Check sheet for the modelled part. Datum: model origin and axes. Units: mm. Give positions to 0.01 mm unless a question says otherwise; leave off trailing zeros. Write each loop counter-clockwise with the first axis right and the second up, starting at its lowest first coordinate (ties: lowest second). Pieces come first, ordered by that corner, then holes.
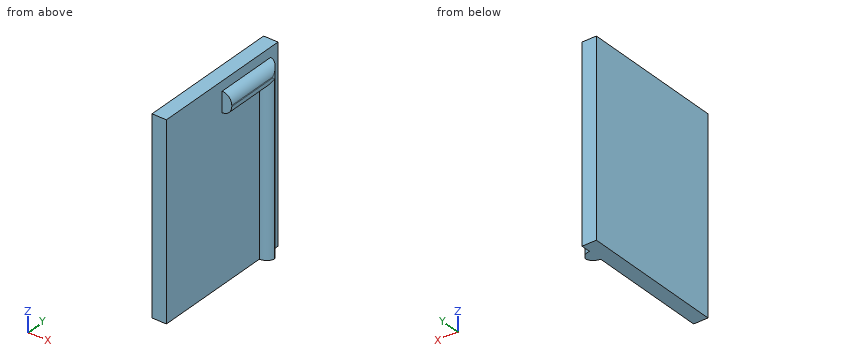
from build123d import *

# Parameters (mm, degrees)
SKETCH1_W           = 40
SKETCH1_H           = 30
BOSS_EXTRUDE1_DEPTH = 3
BOSS_EXTRUDE2_DEPTH = 2
FILLET1_R           = 2


with BuildPart() as part:
    # Sketch1 → Boss-Extrude1 (new body)
    with BuildSketch(Plane(origin=(0, 0, 0), x_dir=(0, 0, -1), z_dir=(1, 0, 0))):
        Rectangle(SKETCH1_W, SKETCH1_H)
    extrude(amount=BOSS_EXTRUDE1_DEPTH)

    # Sketch2 → Boss-Extrude2 (add)
    with BuildSketch(Plane(origin=(3, 0, 0), x_dir=(0, 0, -1), z_dir=(1, 0, 0))):
        Polygon((20, 10), (20, 13), (-13.768503326, 13), (-18, 13), (-18, 10), (-18, 0), (-13.768503326, 0), (-13.768503326, 10), align=None)
    extrude(amount=BOSS_EXTRUDE2_DEPTH)

    # Fillet1
    # the kernel refuses this fillet: 2 mm, written as the material it takes off along each edge
    with BuildSketch(Plane(origin=(5, -5, 18), x_dir=(-1, 0, 0), z_dir=(0, 1, 0))) as fillet1_piece_1:
        with BuildLine():
            CenterArc((FILLET1_R, -FILLET1_R), FILLET1_R, 90, 90)
            Line((0, -FILLET1_R), (0, 0))
            Line((0, 0), (FILLET1_R, 0))
        make_face()
    extrude(amount=23, mode=Mode.SUBTRACT)
    with BuildSketch(Plane(origin=(5, -5, 13.768503326), x_dir=(-1, 0, 0), z_dir=(0, 1, 0))) as fillet1_piece_2:
        with BuildLine():
            CenterArc((FILLET1_R, FILLET1_R), FILLET1_R, 180, 90)
            Line((0, FILLET1_R), (0, 0))
            Line((0, 0), (FILLET1_R, 0))
        make_face()
    extrude(amount=15, mode=Mode.SUBTRACT)
    with BuildSketch(Plane(origin=(5, 10, 13.768503326), x_dir=(-1, 0, 0), z_dir=(0, 0, -1))) as fillet1_piece_3:
        with BuildLine():
            CenterArc((FILLET1_R, FILLET1_R), FILLET1_R, 180, 90)
            Line((0, FILLET1_R), (0, 0))
            Line((0, 0), (FILLET1_R, 0))
        make_face()
    extrude(amount=38.768503326, mode=Mode.SUBTRACT)
    with BuildSketch(Plane(origin=(5, 13, 23), x_dir=(-1, 0, 0), z_dir=(0, 0, -1))) as fillet1_piece_4:
        with BuildLine():
            CenterArc((FILLET1_R, -FILLET1_R), FILLET1_R, 90, 90)
            Line((0, -FILLET1_R), (0, 0))
            Line((0, 0), (FILLET1_R, 0))
        make_face()
    extrude(amount=48, mode=Mode.SUBTRACT)
    with BuildSketch(Plane(origin=(5, 10, 18.768503326), x_dir=(-1, 0, 0), z_dir=(0, 0, -1))) as fillet1_piece_5a_section:
        with BuildLine():
            CenterArc((FILLET1_R, FILLET1_R), FILLET1_R, 180, 90)
            Line((0, FILLET1_R), (0, 0))
            Line((0, 0), (FILLET1_R, 0))
        make_face()
    fillet1_piece_5a = extrude(amount=43.768503326, mode=Mode.PRIVATE)
    fillet1_piece_5a = split(fillet1_piece_5a, bisect_by=Plane(origin=(4.547209771, 10.452790229, 13.768503326), z_dir=(0, 0, 1)), keep=Keep.TOP, mode=Mode.PRIVATE)
    with BuildSketch(Plane(origin=(5, -5, 13.768503326), x_dir=(-1, 0, 0), z_dir=(0, 1, 0))) as fillet1_piece_5b_section:
        with BuildLine():
            CenterArc((FILLET1_R, FILLET1_R), FILLET1_R, 180, 90)
            Line((0, FILLET1_R), (0, 0))
            Line((0, 0), (FILLET1_R, 0))
        make_face()
    fillet1_piece_5b = extrude(amount=20, mode=Mode.PRIVATE)
    fillet1_piece_5b = split(fillet1_piece_5b, bisect_by=Plane(origin=(4.547209771, 10, 14.221293555), z_dir=(0, 1, 0)), keep=Keep.TOP, mode=Mode.PRIVATE)
    fillet1_piece_5 = fillet1_piece_5a & fillet1_piece_5b
    add(fillet1_piece_5, mode=Mode.SUBTRACT)


solid = part.part
1) Scan lines: L1, parallel to X at y = 7.5, z = 3; L2, parallel to Y at x = 3.25, z = 1.5; L3, parallel to Z at x = 3.8, y = 2.25. Record each from-to range of solid material in increasing order.
2) Gauge pin test, flat ends, axial feed: pin 1 (6 mm diameter, centred on y = -4.5, z = -16, fed in from +X); pin 2 (1.5 mm diameter, centred on x = 4, z = -6.5, fed in from +Y); pin 3 (15 mm diameter, centred on y = 3, z = 7.5, fed in from +X). Record the tip position at first contact, or that the pin passes through.
3) Sectioned sample at B-B on y = 6. Record the boundary of the cut face in (x, z), then the cut area to 3 significant figures.
4) Sectioned sample at D-D on y = -1. Record the boundary of the cut face in (x, z), then the cut area to 3 significant figures.
5) Sectioned sample at A-A on z = 5. Record the boundary of the cut face in (x, y).
6) Sectioned sample at C-C on x = 4.3. Record the boundary of the cut face in (y, z), then the cut area to 3 significant figures.
Answers below:
1. L1: x = 0 to 3
1. L2: y = 10.02 to 12.98
1. L3: z = 13.94 to 17.83
2. pin 1: stops at x = 3
2. pin 2: stops at y = 12.98
2. pin 3: stops at x = 4.85
3. outline: (0, -20) - (3, -20) - (3, 13.77) arc R2 ccw to (5, 15.77) - (5, 16) arc R2 ccw to (3, 18) - (3, 20) - (0, 20) - close
3. area: 127 mm2
4. outline: (0, -20) - (3, -20) - (3, 20) - (0, 20) - close
4. area: 120 mm2
5. outline: (0, -15) - (3, -15) - (3, 10) arc R2 ccw to (4.94, 11.5) arc R2 ccw to (3, 13) - (3, 15) - (0, 15) - close
6. outline: (0, 14.25) - (10.48, 14.25) - (10.48, -20) - (12.52, -20) - (12.52, 17.52) - (0, 17.52) - close
6. area: 111 mm2
